Can you work these out from the model? Positions are in its coordinate system, mm. A direction names the side the tool comes from. Round coordinates to 2 decimals unless told otherwise and drop trailing zeros. Loops run counter-clockwise (first coordinate to the right, second up) from the corner with the lowest first, then second, coordinate; pieces in that order, holes last. Notation, with made-up numbers: (23.25, 74) -> (27.25, 74) arc R30 cw to (27.25, 112) -> close; hole circle Ø9 at (36.5, -23.75). An arc over 180 degrees is marked (long way). Write item = value, one per line.
Autodesk Inventor part; units mm, degrees
ref_plane "Work Plane1" through (8, 0, 0) normal (0, 0, -1) x (1, 0, 0)
ref_plane "YZ Plane" through (0, 0, 0) normal (1, 0, 0) x (0, 1, 0)
ref_plane "XZ Plane" through (0, 0, 0) normal (0, 1, 0) x (-1, 0, 0)
sketch "Skizze1" plane through (0, 0, 0) normal (0, 0, 1) x (1, 0, 0)
  line L0 (0, 0) -> (10.5, 0)
  line L1 (10.5, 0) -> (10.5, 1.5)
  line L2 (10.5, 1.5) -> (6, 1.5)
  line L3 (6, 1.5) -> (6, 2)
  line L4 (6, 2) -> (0, 2)
  line L5 (0, 2) -> (0, 0)
  line L6 (-2.1, 0) -> (12.6, 0)
  line L7 (0, -0.4) -> (0, 2.4)
  arc A0 (6, 1.5) -> (6.5, 1.5) centre (6.25, 1.933) ccw
  dimension "d0" = 6
  dimension "d1" = 4.5
  dimension "d2" = 3
  dimension "d3" = 4
  dimension "d14" = 0.5
  dimension "d15" = 0.5
revolve "Körper" add sketch "Skizze1" angle 360 about axis through (0, 0, 0) along (1, 0, 0)
sketch "Skizze2" plane through (0, 0, 0) normal (-1, 0, 0) x (0, 0, 1)
  circle A0 centre (0, 0) radius 2
  line L0 (0, -2.8) -> (0, 2.8)
  line L1 (-2.8, 0) -> (2.8, 0)
  line L2 (-2, 0.25) -> (2, 0.25)
  line L3 (2, 0.25) -> (2, -0.25)
  line L4 (2, -0.25) -> (-2, -0.25)
  line L5 (-2, -0.25) -> (-2, 0.25)
  line L6 (-2, 0) -> (2, 0) construction
  line L7 (0, 0.25) -> (0, -0.25) construction
  dimension "d5" = 0.5
extrude "Loch" cut sketch "Skizze2" against normal blind 1.05 contours L1 L0 L2 A0 | L3 L4 A0 | A0 L4 L0 L1 | A0 L2 L3 | L1 A0 L2 L0 | L0 L4 A0 L1 | L5 L2 A0 | A0 L4 L5
chamfer "Fase1" distance 0.5 angle 45 3 edges at (0, 1.5, -1.3229) (0, 1.5, 1.3229) (0, -2, 0) measured on face at (4, -0.8596, 1.8058)
thread "Gewinde"
chamfer "Fase2" distance 0.3067 distance2 0.3067 1 edges at (10.5, -1.5, 0) measured on face at (10.5, -0.533, -0.3123)
revolve "Nut1" cut sketch "Skizze1" angle 360 about axis through (0, 0, 0) along (1, 0, 0) contours A0 L2
ref_plane "Work Plane1" through (8, 0, 0) normal (0, 0, -1) x (1, 0, 0)
equation "\"d0\" = KOH"
equation "\"d1\" = GEL"
equation "\"d2\" = NND"
equation "\"d3\" = KOD"
equation "\"d14\" = SBR"
equation "\"d15\" = SBR"
equation "\"d5\" = SBR"
equation "\"d6\" = STI"
equation "\"d8\" = PHH"
equation "\"d19\" = PHH"
equation "\"d10\" = GEL"
equation "\"d12\" = -0.5 * GD1 + 0.5 * NND"
equation "\"d13\" = GUL"
equation "\"NND\" = 3"
equation "\"GEL\" = 4.5"
equation "\"KOD\" = 4"
equation "\"KOH\" = 6"
equation "\"SBR\" = 0.5"
equation "\"GUL\" = 0.61345 * PTC"
equation "\"PHH\" = 0.5"
equation "\"GD1\" = THREADDIA - 1.2269 * PTC"
equation "\"STI\" = 1.05"
equation "\"THREADDIA\" = 3"
equation "\"TOA\" = 30deg"
equation "\"NLG\" = GEL"
equation "\"PTC\" = 0.5"
equation "\"GAL\" = 0.61345 * PTC"
properties part number "DIN 927 - M3 x 6-14H" material "Stahl, weich"
1. I need wall thicknesses on line 1 (Y direction, x = 2, z = 0.1); line 2 (Y direction, x = 1, z = 1.15); line 3 (Y direction, x = 4.75, z = -1.4). Which ranges of each line are inside material? Lowest first, please. Write a range as [from, to].
Entries:
line_1 = [-2, 2]
line_2 = [-1.64, -0.25], [0.25, 1.64]
line_3 = [-1.43, 1.43]
2. Suppose I cut it at B-B, the plane z = 0. List the corners of the cut face in (x, y) for me, and give its area (3 significant figures).
Entries:
outline = (0, -1.5) -> (0.5, -2) -> (6, -2) -> (6, -1.5) arc R0.5 cw to (6.5, -1.5) -> (10.19, -1.5) -> (10.5, -1.19) -> (10.5, 1.19) -> (10.19, 1.5) -> (6.5, 1.5) arc R0.5 cw to (6, 1.5) -> (6, 2) -> (0.5, 2) -> (0, 1.5) -> (0, 0.25) -> (1.05, 0.25) -> (1.05, -0.25) -> (0, -0.25) -> close
area = 36.6 mm²
3. I'm going to push flat-ended pins straight in: pin 1 (0.8 mm diameter, centred on x = 0.5, z = 0.5, fed in from +Y); pin 2 (1.2 mm diameter, centred on x = 0.5, z = 1, fed in from -Y); pin 3 (1 mm diameter, centred on x = 3, z = 1, fed in from -Y). Where does each tip first touch, or does it pass through?
Entries:
pin_1 = 2
pin_2 = -1.96
pin_3 = -1.94
4. Suppose I cut it at A-A, the plane y = 0. List the corners of the cut face in (x, z) for me.
Entries:
outline = (1.05, -2) -> (6, -2) -> (6, -1.5) arc R0.5 cw to (6.5, -1.5) -> (10.19, -1.5) -> (10.5, -1.19) -> (10.5, 1.19) -> (10.19, 1.5) -> (6.5, 1.5) arc R0.5 cw to (6, 1.5) -> (6, 2) -> (1.05, 2) -> close
5. For faces 1 (the flat face through (0.5, 0.25, 0)), 2 (the conical face through (0.14, 1.64, -0.03)), 3 (the cylindrical face through (8.32, -1.5, -0.07)), which set-ups out of +Z, -Z, +X, -X, +Y, -Y let a thin tool reach every point of the face, with its end or its side?
Entries:
face_1 = +Z, -Z, -X
face_2 = -X, +Y
face_3 = +X
